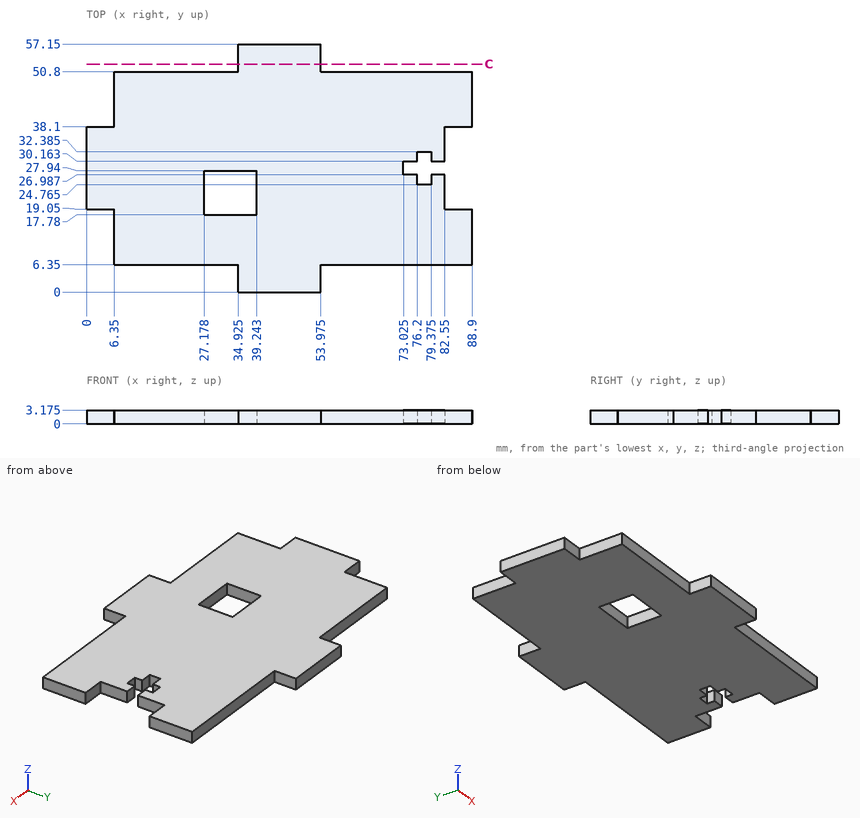
Geometry check sheet. Reference: drawing and pictorial views, mm from the part's lowest x, y, z. Give positions to 0.01 mm unless a question says otherwise; leave off trailing zeros. Loops run counter-clockwise (first coordinate to the right, second up) from the corner with the lowest first, then second, coordinate; pieces in that order, holes last. Notation, with made-up numbers: (-3, 18) -> (39, 18) arc R25 ccw to (39, 41) -> close; hole circle Ø1 at (22, -21). An arc over 180 degrees is marked (long way). Answer in a Markdown table with one row per item. Add a question column.
1) Cross-section at C-C on y = 52.5. Record the boundary of the cut face in (x, z) (1 decimal).
2) Gauge pin test, flat ends, axial feed: P1, Ø1, axis at x = 77.5, z = 1.5, coming from the +Y side; P2, Ø1.6, axis at y = 3.5, z = 1, coming from the +X side (1 decimal); P3, Ø1, axis at x = 74.5, z = 2, coming from the -Y side. Record the tip position at first contact, or that the pin passes through.
3) Material ranges on probe 1 along Y at (x, z) = (31, 0.95); probe 2 along X at (y, z) = (19, 1.95); probe 3 along X at (y, z) = (21.5, 2.7), recorded low to high. Write a range as from..to.
Outcome:
| question | item | result |
|---|---|---|
| 1 | outline | (34.9, 0) -> (54, 0) -> (54, 3.2) -> (34.9, 3.2) -> close |
| 2 | P1 | stops at y = 50.8 |
| 2 | P2 | stops at x = 54 |
| 2 | P3 | stops at y = 6.35 |
| 3 | probe 1 | y = 6.35..17.78, 27.94..50.8 |
| 3 | probe 2 | x = 6.35..27.18, 39.24..88.9 |
| 3 | probe 3 | x = 0..27.18, 39.24..82.55 |
